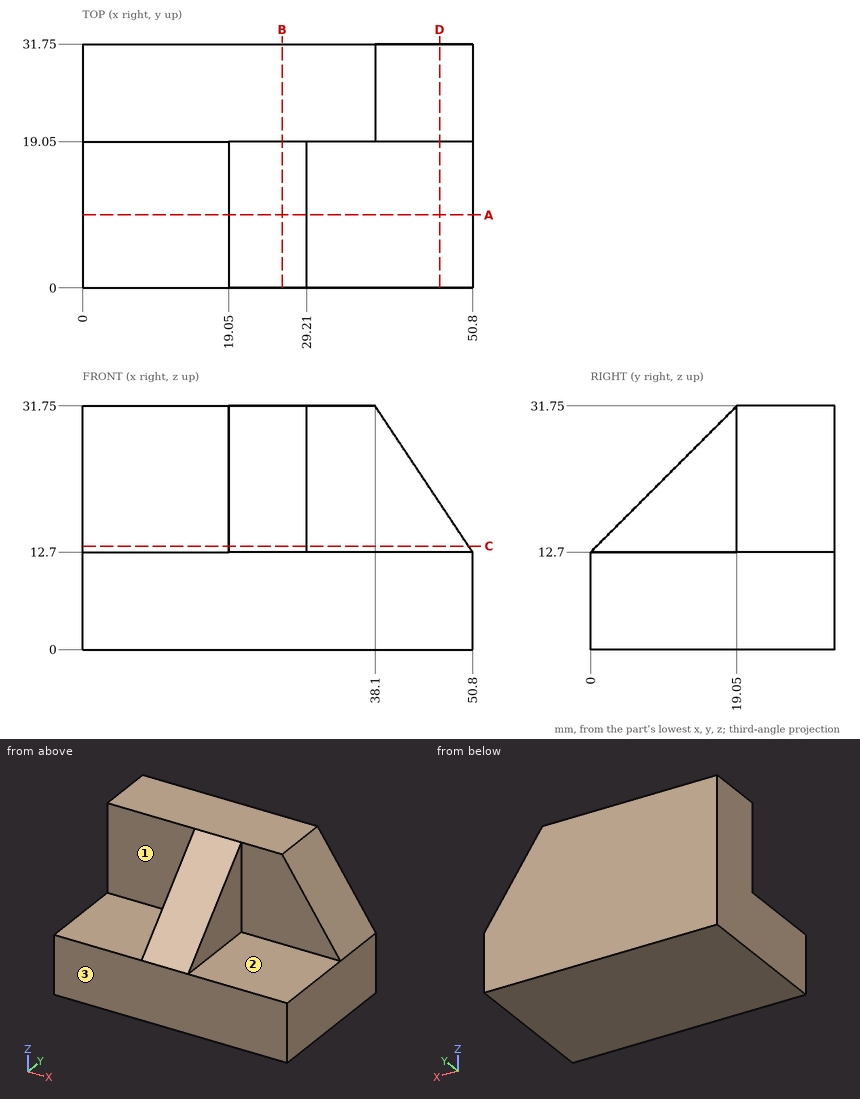
The drawing under review shows one solid part. Ordinate dimensions are in mm from its lowest x, y, z. A direction names the side the tool comes from. Give positions to 0.01 mm unless a question says otherwise; leave off trailing zeros. Order: outer loops, then holes, each group sorted by start corner. A loop starts at its lowest first (then second) coordinate and runs counter-clockwise, first axis right, second up. Notation, with made-up numbers: M -31.75,0.25 L -26.75,0.25 A20 ccw -26.75,16.25 Z; hole C -7.75,34 d11. An arc over 180 degrees is marked long. One line per question, with ' | ' between items. Start each with the question number.
Q1. We need section B-B (x = 26). Write out the cut boundary in (y, z), plus the area to 3 significant figures.
Q2. For pin 1 Ø9.5 at (x, y) = (44, 8.5) entering from +Z; pin 2 Ø9.5 at (y, z) = (12.5, 20) entering from -X; pin 3 Ø15 at (x, z) = (38.5, 20.5) entering from -Y, all flat-tipped, find the tip position at first contact; note any pin that passes through.
Q3. We need section D-D (x = 46.5). Write out the cut boundary in (y, z).
Q4. Machinability: for the marked faces 1, 2 and 3, which of the approach directions +Z, -Z, +X, -X, +Y, -Y give a long, thin tool a straight path to every point of the face, cutting with its end or side? Answer none if there is none.
Q5. For L1, parallel to Z at x = 4.5, y = 16.5; L2, parallel to Y at x = 4, z = 23; L3, parallel to X at y = 10.5, z = 21.5, list the stretches that pass through material, from the lowest coordinate up. Write a range as [from, to].
Q6. We need section A-A (y = 9.5). Write out the cut boundary in (x, z).
Q7. We need section C-C (z = 13.5). Write out the cut boundary in (x, y).
Returned:
1) outline: M 0,0 L 31.75,0 L 31.75,31.75 L 19.05,31.75 L 0,12.7 Z | area: 827 mm2
2) pin 1: z = 12.7 | pin 2: x = 19.05 | pin 3: y = 19.05
3) outline: M 0,0 L 31.75,0 L 31.75,19.15 L 19.05,19.15 L 19.05,12.7 L 0,12.7 Z
4) face 1: +Z, -X, -Y | face 2: +Z, +X, -Y | face 3: +Z, -Z, +X, -X, -Y
5) L1: [0, 12.7] | L2: [19.05, 31.75] | L3: [19.05, 29.21]
6) outline: M 0,0 L 50.8,0 L 50.8,12.7 L 29.21,12.7 L 29.21,22.2 L 19.05,22.2 L 19.05,12.7 L 0,12.7 Z
7) outline: M 0,19.05 L 19.05,19.05 L 19.05,0.8 L 29.21,0.8 L 29.21,19.05 L 50.27,19.05 L 50.27,31.75 L 0,31.75 Z
